Geometry check sheet. Reference: the model listing, model coordinates, mm. Give positions to 0.01 mm unless a question says otherwise; leave off trailing zeros. Loops run counter-clockwise (first coordinate to the right, second up) from the corner with the lowest first, then second, coordinate; pieces in that order, holes last.
```python
from build123d import *

# Parameters (mm, degrees)
SKETCH_1_R      = 2
EXTRUDE_1_DEPTH = 3


with BuildPart() as part:
    # 草图1 → 凸台-拉伸1 (new body)
    with BuildSketch(Plane(origin=(0, 0, 0), x_dir=(1, 0, 0), z_dir=(0, 1, 0))):
        with BuildLine():
            Line((-5.337642525, 6.81342157), (4.662357475, 24.133929646))
            Line((4.662357475, 24.133929646), (-29.978658676, 44.133929646))
            Line((-29.978658676, 44.133929646), (-39.978658676, 26.81342157))
            ThreePointArc((-39.978658676, 26.81342157), (-40.718178371, 11.008358068), (-46.138912714, -3.856451411))
            Line((-46.138912714, -3.856451411), (-28.818404638, -13.856451411))
            ThreePointArc((-28.818404638, -13.856451411), (-18.655469178, -1.729553023), (-5.337642525, 6.81342157))
        make_face()
        with Locations(Location((-26.318404638, 30.473675608, 0), (0, 0, 270))):
            Circle(SKETCH_1_R, mode=Mode.SUBTRACT)
        with Locations(Location((-17.713393416, 25.377992244, 0), (0, 0, 270))):
            Circle(SKETCH_1_R, mode=Mode.SUBTRACT)
        with Locations(Location((-8.997896563, 20.473675608, 0), (0, 0, 270))):
            Circle(SKETCH_1_R, mode=Mode.SUBTRACT)
        with Locations(Location((-27.533901492, 8.368373301, 0), (0, 0, 270))):
            Circle(SKETCH_1_R, mode=Mode.SUBTRACT)
        with Locations(Location((-32.478658676, -0.196197373, 0), (0, 0, 270))):
            Circle(SKETCH_1_R, mode=Mode.SUBTRACT)
    extrude(amount=EXTRUDE_1_DEPTH)


solid = part.part
```
1) Scan lines: line 1 along Z through (x, y) = (-28.5, 1.2); line 2 along Z through (x, y) = (-19.5, 1.55); line 3 along X through (y, z) = (1.15, 9.5). Record each from-to range of solid material in increasing order.
2) Mould release check, pull along X, two halves, no side actions. Record for faces 1 (the cylindrical face through (-26.23, 1.48, -32.47)), 2 (the flat face through (-21, 3, -16)), 3 (the cylindrical face through (-40.675, 1.479, -11.226)): +X half, -X half, draft (parallel to the pull), parting line (faces both ways), or undercut.
3) Sectioned sample at C-C on z = -38. Enter the section's corners in (x, y), plus the area to 3 significant figures.
4) Sectioned sample at D-D on x = 1.5. Enter the section's corners in (y, z), plus the area to 3 significant figures.
5) Sectioned sample at A-A on y = 1. Enter the section's corners in (x, z), plus the area to 3 significant figures.
6) Sectioned sample at B-B on x = -8. Enter the section's corners in (y, z).
Determined:
1. line 1: z = -43.28 to -10.12, -6.62 to 13.34
1. line 2: z = -38.08 to -26.28, -24.48 to 2.49
1. line 3: x = -36.36 to -25.86
2. face 1: undercut
2. face 2: draft
2. face 3: -X half
3. outline: (-33.52, 0) - (-19.35, 0) - (-19.35, 3) - (-33.52, 3) - close
3. area: 42.5 mm2
4. outline: (0, -25.96) - (3, -25.96) - (3, -18.66) - (0, -18.66) - close
4. area: 21.9 mm2
5. outline: (-46.14, 3.86) arc R52.43 cw to (-39.98, -26.81) - (-29.98, -44.13) - (4.66, -24.13) - (-5.34, -6.81) arc R52.43 cw to (-28.82, 13.86) - close; hole circle Ø4 at (-32.48, 0.2); hole circle Ø4 at (-27.53, -8.37); hole circle Ø4 at (-26.32, -30.47); hole circle Ø4 at (-17.71, -25.38); hole circle Ø4 at (-9, -20.47)
5. area: 1,530 mm2
6. outline: (0, -31.44) - (3, -31.44) - (3, -22.21) - (0, -22.21) - close; (0, -18.74) - (3, -18.74) - (3, -5.54) - (0, -5.54) - close
